from build123d import *

# Parameters (mm, degrees)
F0_R      = 102
F0_R_2    = 100
F1_DEPTH  = 250
F2_R      = 127
F2_R_2    = 102
F2_R_3    = 100
F3_DEPTH  = 25
F4_R      = 102
F4_R_2    = 100
F5_DEPTH  = 25
F7_D      = 8.4
F8_R      = 50
F9_DEPTH  = 300.001
F10_D     = 8.4
F10_DEPTH = 9
F10_TIP   = 2.5236145999


with BuildPart() as f1:
    # F0 (on Front) → F1 (new body)
    with BuildSketch(Plane.XZ):
        Circle(F0_R)
        Circle(F0_R_2, mode=Mode.SUBTRACT)
    extrude(amount=F1_DEPTH)

    # F2 (on face) → F3 (join)
    with BuildSketch(Plane.XZ.offset(250)):
        Circle(F2_R)
        Circle(F2_R_2, mode=Mode.SUBTRACT)
        Circle(F2_R_2)
        Circle(F2_R_3, mode=Mode.SUBTRACT)
    extrude(amount=F3_DEPTH)

    # F4 (on face) → F5 (join)
    with BuildSketch(Plane(origin=(0, 0, 0), x_dir=(-1, 0, 0), z_dir=(0, 1, 0))):
        Circle(F4_R)
        Circle(F4_R_2, mode=Mode.SUBTRACT)
        Circle(F4_R_2)
    extrude(amount=F5_DEPTH)

    # F7 (through all)
    with Locations(Plane.XZ.offset(275)):
        with Locations((0, 116), (30.0230092319, 112.0473958495), (58, 100.458946839), (82.0243866176, 82.0243866176), (100.458946839, 58), (112.0473958495, 30.0230092319), (116, 0), (112.0473958495, -30.0230092319), (100.458946839, -58), (82.0243866176, -82.0243866176), (58, -100.458946839), (30.0230092319, -112.0473958495), (0, -116), (-30.0230092319, -112.0473958495), (-58, -100.458946839), (-82.0243866176, -82.0243866176), (-100.458946839, -58), (-112.0473958495, -30.0230092319), (-116, 0), (-112.0473958495, 30.0230092319), (-100.458946839, 58), (-82.0243866176, 82.0243866176), (-58, 100.458946839), (-30.0230092319, 112.0473958495)):
            Hole(F7_D / 2)

    # F8 (on face) → F9 (cut, through all)
    with BuildSketch(Plane(origin=(0, 25, 0), x_dir=(-1, 0, 0), z_dir=(0, 1, 0))):
        with Locations((5, 22.5)):
            Circle(F8_R)
    extrude(amount=-F9_DEPTH, mode=Mode.SUBTRACT)

    # F10
    with Locations(Plane(origin=(0, 25, 0), x_dir=(-1, 0, 0), z_dir=(0, 1, 0))):
        with Locations((5, 87.5), (-19.8744231037, -37.5521696132), (-40.9619407771, -23.4619407771), (-55.0521696132, -2.3744231037), (-60, 22.5), (-55.0521696132, 47.3744231037), (-40.9619407771, 68.4619407771), (-19.8744231037, 82.5521696132), (29.8744231037, 82.5521696132), (50.9619407771, 68.4619407771), (65.0521696132, 47.3744231037), (70, 22.5), (65.0521696132, -2.3744231037), (50.9619407771, -23.4619407771), (29.8744231037, -37.5521696132), (5, -42.5)):
            Hole(F10_D / 2, depth=F10_DEPTH)
            with Locations((0, 0, -(F10_DEPTH + F10_TIP / 2))):  # 118° drill point
                Cone(0, F10_D / 2, F10_TIP, mode=Mode.SUBTRACT)


solid = f1.part
The listing builds one solid part. Answer for the finished solid, in the listing's coordinates (mm). A direction names the side the tool comes from. Coordinates: 2 decimals unless noted, no trailing zeros. Write each loop counter-clockwise with the first axis right and the second up, starting at its lowest first coordinate (ties: lowest second). Pieces come first, ordered by that corner, then holes. Notation, with made-up numbers: M 78.5,84 L 86.5,84 A14 cw 86.5,98 Z; hole C -14,-3 d6. An arc over 180 degrees is marked long. Write each question's results on one line, items separated by ' | '.
Item 1: Given P1, Ø9.5, axis at x = -30.02, z = 112.05, coming from the +Y side; P2, Ø7.5, axis at x = -116, z = 0, coming from the +Y side; P3, Ø2, axis at y = -199, z = -63.5, coming from the +X side; P4, Ø8, axis at y = -23, z = -29.5, coming from the -X side, each flat-ended and moving along its own axis, determine where each tip first touches the part or whether it passes through.
Answer below:
P1: y = -250 | P2: through | P3: x = 80.61 | P4: x = -98.76
Item 2: The part is cut by section C-C on z = -58. Determine the outline of the cut face in (x, y), and give its area (3 significant figures).
Answer below:
outline: M -112.98,-275 L -104.66,-275 L -104.66,-250 L -112.98,-250 Z; M -96.26,-275 L -81.46,-275 L -81.46,0 L 81.46,0 L 81.46,-275 L 96.26,-275 L 96.26,-250 L 83.9,-250 L 83.9,25 L -83.9,25 L -83.9,-250 L -96.26,-250 Z; M 104.66,-275 L 112.98,-275 L 112.98,-250 L 104.66,-250 Z | area: 6,570 mm2
Item 3: The part is cut by section A-A on z = 13. Determine the outline of the cut face in (x, y), and give its area (3 significant figures).
Answer below:
outline: M -126.33,-275 L -99.15,-275 L -99.15,0 L -54.09,0 L -54.09,25 L -101.17,25 L -101.17,-250 L -126.33,-250 Z; M 44.09,0 L 99.15,0 L 99.15,-275 L 126.33,-275 L 126.33,-250 L 101.17,-250 L 101.17,25 L 44.09,25 Z | area: 4,970 mm2
Item 4: The part is cut by section B-B on y = -54. Determine the outline of the cut face in (x, z), and give its area (3 significant figures).
Answer below:
outline: C 0,0 d204; hole C 0,0 d200 | area: 1,270 mm2
Item 5: Which of the six approach directions +Z, -Z, +X, -X, +Y, -Y give full straight-line access (tool end or side, diameter ignored) to faces 1 (the face through (-29.476, -262.325, 116.212)), 2 (the face through (-2.74, 20.44, -38.96)), 3 (the face through (95.38, -135.57, 30.04))?
Answer below:
face 1: +Y, -Y | face 2: +Y | face 3: -Y
Item 6: Consider probe 1 along Z at (x, y) = (0, -256); probe 2 along Z at (x, y) = (2, -135); probe 3 along Y at (x, z) = (-108, 4). Determine where each line is inside the solid, lowest interval first. Write a range as [from, to].
Answer below:
probe 1: [-127, -120.2], [-111.8, -100], [100, 111.8], [120.2, 127] | probe 2: [-101.98, -99.98], [99.98, 101.98] | probe 3: [-275, -250]
